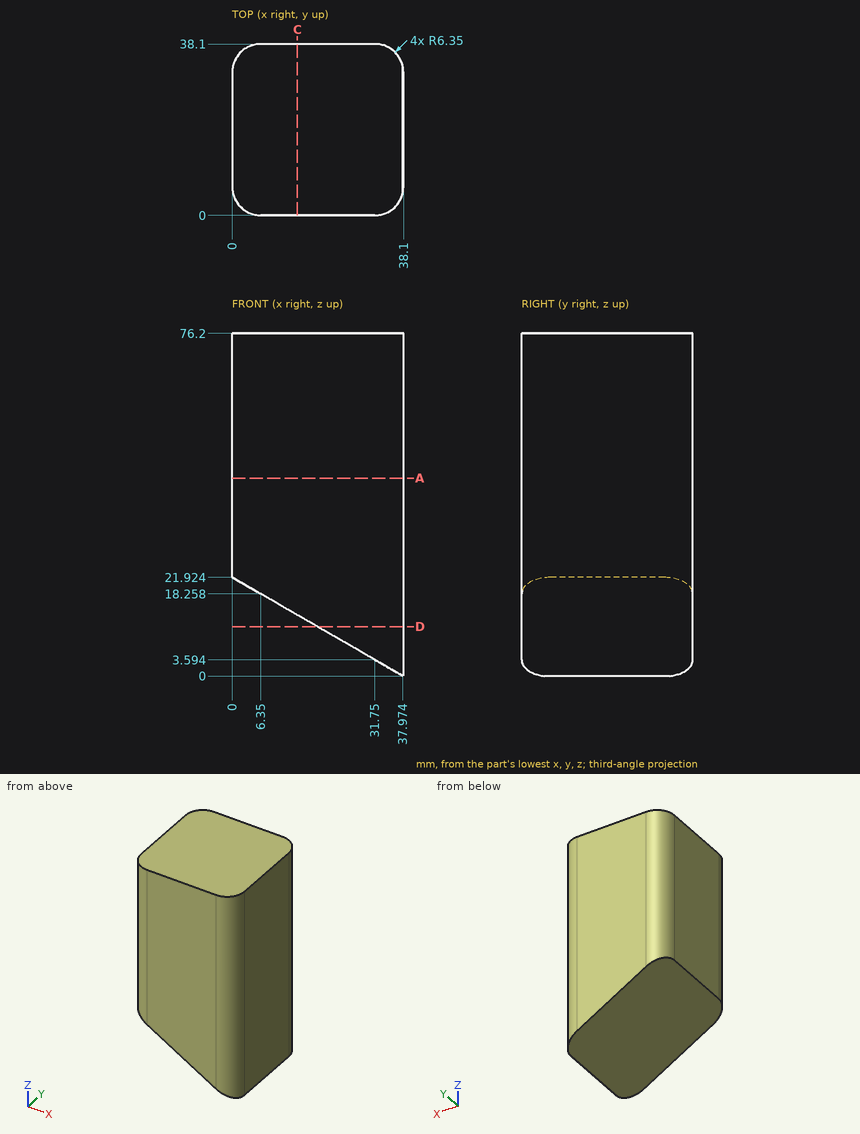
Drawing for the job (mm, zero at the part's lowest x, y, z). Give positions to 0.01 mm unless a question says otherwise; leave off trailing zeros. Order: outer loops, then holes, each group sorted by start corner. A loop starts at its lowest first (then second) coordinate and runs counter-clockwise, first axis right, second up. Notation, with made-up numbers: M 78.25,13 L 100.25,13 A16 ccw 100.25,41 Z; hole C -5.75,-34.75 d7. An arc over 180 degrees is marked long. Write item = value, one per line. Start each with the question number.
(1) Pin check, flat tips, straight feed: pin 1 Ø8 at (x, y) = (7.5, 29) entering from -Z (1 decimal); pin 2 Ø8 at (x, y) = (26, 29.5) entering from -Z (1 decimal). Stop position of each tip, or through.
(2) Probe L1, parallel to Z at x = 18, y = 16.5; L2, parallel to Y at x = 5, z = 49 (1 decimal); L3, parallel to Z at x = 8, y = 34.5 (1 decimal). List the from-to ranges inside material, lowest first. Write a range as [from, to].
(3) Slice it at C-C on x = 14.5. Write the cut outline in (y, z).
(4) Slice it at A-A on z = 44. Write the cut outline in (x, y).
(5) Slice it at D-D on z = 11. Write the cut outline in (x, y), plus the area to 3 significant figures.
Responses:
q1.pin_1 = 15.3
q1.pin_2 = 4.6
q2.L1 = [11.53, 76.2]
q2.L2 = [0.1, 38]
q2.L3 = [17.3, 76.2]
q3.outline = M 0,13.55 L 38.1,13.55 L 38.1,76.2 L 0,76.2 Z
q4.outline = M 0,6.35 A6.35 ccw 6.35,0 L 31.75,0 A6.35 ccw 38.1,6.35 L 38.1,31.75 A6.35 ccw 31.75,38.1 L 6.35,38.1 A6.35 ccw 0,31.75 Z
q5.outline = M 18.92,0 L 31.75,0 A6.35 ccw 38.1,6.35 L 38.1,31.75 A6.35 ccw 31.75,38.1 L 18.92,38.1 Z
q5.area = 713 mm2
